For this review, take the finished solid that the model builds, in its own axes (mm). A direction names the side the tool comes from. Give positions to 0.01 mm unless a question says otherwise; leave off trailing zeros. Loops run counter-clockwise (first coordinate to the right, second up) from the corner with the lowest first, then second, coordinate; pieces in that order, holes last. Notation, with made-up numbers: (85.25, -28) - (105.25, -28) arc R13 ccw to (105.25, -15) - close; hole circle Ø7 at (85, 88). An arc over 180 degrees is marked (long way). Answer in a Markdown table with one row per item.
```python
from build123d import *


with BuildPart() as part:
    # Esquisse1 → Révolution1 (revolve)
    with BuildSketch(Plane.XY, mode=Mode.PRIVATE) as r_volution1_sk:
        Polygon((115, 80.978839747), (250, 80.978839747), (170, 670.978839747), (87.5, 670.978839747), (87.5, 290.978839747), (115, 290.978839747), align=None)
        with BuildLine():
            Line((115, 20.978839747), (320, 20.978839747))
            ThreePointArc((320, 20.978839747), (275.487697577, 39.881153587), (250, 80.978839747))
            Line((250, 80.978839747), (115, 80.978839747))
            Line((115, 80.978839747), (115, 20.978839747))
        make_face()
        Polygon((180, -39.021160253), (180, -79.021160253), (320, -79.021160253), (320, 20.978839747), (115, 20.978839747), (115, -39.021160253), align=None)
    revolve(r_volution1_sk.sketch.rotate(Axis((0, -112.379494544, 0), (0, 1, 0)), 90), axis=Axis((0, -112.379494544, 0), (0, 1, 0)))


solid = part.part
```
1. Mouldability with a two-part tool opening along Z and no side actions: class faces 3 (the face through (-14.07, -28.32, 319.69)), 4 (the face through (138, -79.021, 138)), 5 (the face through (159.69, -59.3, -83.06)) as released by +Z, released by -Z, zero draft, split by the parting line, or undercut.
Values:
| item | result |
|---|---|
| face 3 | split by the parting line |
| face 4 | zero draft |
| face 5 | undercut |
2. We need section C-C, the plane y = 517. Give the boundary of the cut face in (x, z).
Values:
| item | result |
|---|---|
| outline | circle Ø381.76 at (0, 0); hole circle Ø175 at (0, 0) |
3. We need section A-A, the plane z = 0. Give the boundary of the cut face in (x, y), and give its area (3 significant figures).
Values:
| item | result |
|---|---|
| outline | (-320, -79.02) - (-180, -79.02) - (-180, -39.02) - (-115, -39.02) - (-115, 290.98) - (-87.5, 290.98) - (-87.5, 670.98) - (-170, 670.98) - (-250, 80.98) arc R80 cw to (-320, 20.98) - close; (87.5, 290.98) - (115, 290.98) - (115, -39.02) - (180, -39.02) - (180, -79.02) - (320, -79.02) - (320, 20.98) arc R80 cw to (250, 80.98) - (170, 670.98) - (87.5, 670.98) - close |
| area | 187,000 mm^2 |
4. We need section B-B, the plane x = 0. Give the boundary of the cut face in (y, z), and give its area (3 significant figures).
Values:
| item | result |
|---|---|
| outline | (-79.02, -320) - (20.98, -320) arc R80 cw to (80.98, -250) - (670.98, -170) - (670.98, -87.5) - (290.98, -87.5) - (290.98, -115) - (-39.02, -115) - (-39.02, -180) - (-79.02, -180) - close; (-79.02, 180) - (-39.02, 180) - (-39.02, 115) - (290.98, 115) - (290.98, 87.5) - (670.98, 87.5) - (670.98, 170) - (80.98, 250) arc R80 cw to (20.98, 320) - (-79.02, 320) - close |
| area | 187,000 mm^2 |
5. Clearance check with flat-ended pins moving along their axes: pin 1 (1.5 mm diameter, centred on x = 166, z = -39, fed in from -Y); pin 2 (6 mm diameter, centred on x = -91, y = 162.5, fed in from -Z); pin 3 (2 mm diameter, centred on x = 132.5, y = 174, fed in from -Z). State where each tip first meets the part, or that it passes through.
Values:
| item | result |
|---|---|
| pin 1 | stops at y = -39.02 |
| pin 2 | stops at z = -222.23 |
| pin 3 | stops at z = -197.66 |
6. For faces 1 (the face through (112.265, 123.669, 24.93)), 2 (the face through (-86.755, 478.319, 11.391)), list the 3-axis set-ups (+Z, -Z, +X, -X, +Y, -Y) from which the entire face can be reached by the end or side of a thin tool; tool diameter is ignored.
Values:
| item | result |
|---|---|
| face 1 | -Y |
| face 2 | +Y, -Y |
7. Wall thickness on line 1 (X direction, y = -59.5, z = 0); line 2 (X direction, y = 351, z = 37); line 3 (Z direction, x = -97, y = 168.5): over which ranges is each line inside the solid? List them lowest first. Write a range as [from, to].
Values:
| item | result |
|---|---|
| line 1 | x = [-320, -180], [180, 320] |
| line 2 | x = [-210.15, -79.29], [79.29, 210.15] |
| line 3 | z = [-217.48, -61.77], [61.77, 217.48] |
